Autodesk Inventor part; units mm, degrees
ref_plane "YZ Plane" through (0, 0, 0) normal (1, 0, 0) x (0, 1, 0)
ref_plane "XZ Plane" through (0, 0, 0) normal (0, 1, 0) x (-1, 0, 0)
ref_plane "XY Plane" through (0, 0, 0) normal (0, 0, 1) x (1, 0, 0)
sketch "Sketch1" plane through (0, 0, 0) normal (0, 0, 1) x (1, 0, 0)
  circle A0 centre (-48.3826, -94.0192) radius 2.5
  circle A1 centre (2.8152, 8.6005) radius 2.5
  line L0 (-48.3826, -94.0192) -> (40.5013, 54.4144)
  line L1 (2.8152, 8.6005) -> (32.8522, -42.034)
  line L2 (-2.0828, 38.9998) -> (-2.0828, -39)
  line L3 (-2.0828, -0.0001) -> (69.8745, -0.0001)
  line L4 (7.9172, -0.0001) -> (-0.6834, -5.1021)
  line L5 (2.8152, 8.6005) -> (7.9172, -0.0001)
  line L6 (7.9172, -0.0001) -> (16.5177, 5.1019)
  line L7 (7.9172, -0.0001) -> (-0.6834, -5.1021)
  line L8 (-0.6834, -5.1021) -> (-0.6834, -5.1021)
  line L9 (7.9172, -0.0001) -> (16.5177, 5.1019)
  line L10 (16.5177, 5.1019) -> (16.5177, 5.1019)
  line L11 (7.9172, -0.0001) -> (-0.6622, 5.1374)
  line L12 (7.9172, -0.0001) -> (16.4966, -5.1375)
  line L13 (-48.3826, -94.0192) -> (-43.2452, -85.4397)
  line L14 (-54.6233, -56.9895) -> (-9.7188, -83.8789)
  line L15 (-43.2452, -85.4397) -> (-34.6657, -90.5772)
  line L16 (-43.2452, -85.4397) -> (-51.8246, -80.3023)
  line L17 (-34.6657, -90.5772) -> (16.4966, -5.1375)
  line L18 (-0.6622, 5.1374) -> (-51.8246, -80.3023)
  line L19 (-3.7386, 0) -> (13.452, 10.2217)
  line L20 (-3.7386, 0) -> (13.4203, -10.2749)
  circle A2 centre (6.9172, -34) radius 2.5
  circle A3 centre (6.9172, -34) radius 5
  circle A4 centre (6.9172, 34) radius 2.5
  circle A5 centre (6.9172, 34) radius 4.9998
  line L21 (15.8878, 38.9998) -> (-2.0828, 38.9998)
  line L22 (-2.0828, -39) -> (15.933, -39)
  line L23 (-13.3434, -16.0398) -> (19.6624, -35.8041)
  line L24 (-13.3434, 16.0396) -> (19.6624, 35.8039)
  line L25 (-13.3434, -16.0398) -> (-15.9172, -14.4985)
  line L26 (-2.0828, -0.0001) -> (-26.2435, -0.0001)
  line L27 (-15.9172, -14.4985) -> (-7.2354, -0.0001)
  line L28 (-13.3434, 16.0396) -> (-15.9172, 14.4984)
  line L29 (-15.9172, 14.4984) -> (-7.2354, -0.0001)
  line L30 (13.4203, -10.2749) -> (15.9172, -11.7701)
  line L31 (15.933, -39) -> (15.8878, 38.9998)
  line L32 (13.452, 10.2217) -> (15.9037, 11.6795)
  line L33 (15.9037, 11.6795) -> (6.3124, 27.8097)
  line L34 (15.9172, -11.7701) -> (6.3124, -27.8099)
  line L35 (15.9037, 11.6795) -> (15.9172, -11.7701)
  line L36 (-15.9172, -14.4985) -> (-15.9172, 14.4984)
  line L37 (6.3124, 27.8097) -> (-15.9172, 14.4984)
  circle A6 centre (-48.3826, -94.0192) radius 2.5
  line L38 (-311.4249, 0) -> (127.5863, 0)
  line L39 (-170.3704, -117.2696) -> (-13.4682, 154.4931)
  line L40 (-102.6648, 0) -> (-157.9558, -95.7668)
  line L41 (-157.9558, -95.7668) -> (-48.3826, -94.0192)
  line L42 (-48.3826, -94.0192) -> (-58.3814, -94.1786)
  line L43 (-58.3814, -94.1786) -> (-58.5408, -84.1799)
  line L44 (-58.5408, -84.1799) -> (-58.2219, -104.1774)
  line L45 (-51.8246, -80.3023) -> (-41.5497, -63.1434)
  line L46 (-41.5497, -63.1434) -> (-24.3908, -73.4184)
  line L47 (-58.5408, -84.1799) -> (-78.5383, -84.4989)
  line L48 (-78.5383, -84.4989) -> (-78.2193, -104.4963)
  line L49 (-78.2193, -104.4963) -> (-58.2219, -104.1774)
  line L50 (-58.5408, -84.1799) -> (-51.8246, -80.3023)
  line L51 (-58.2219, -104.1774) -> (-26.2433, -104.1774)
  line L52 (-34.6657, -90.5772) -> (-48.6317, -113.8999)
  circle A7 centre (-48.3828, -94.0194) radius 2.5
  point P0 (0, 0)
  point P1 (6.9172, -21)
  point P2 (-3.7386, 0)
  point P3 (-42.2878, -64.3761)
  point P4 (-42.8097, -104.1774)
  point P5 (-25.129, -74.6511)
  dimension "d0" = 10
  dimension "d1" = 10
  dimension "d2" = 10
  dimension "d3" = 10
  dimension "d4" = 10
  dimension "d5" = 10
  dimension "d6" = 10
  dimension "d7" = 10
  dimension "d8" = 10
  dimension "d9" = 10
  dimension "d10" = 10
  dimension "d11" = 20
  dimension "d12" = 20
  dimension "d13" = 3
  dimension "d14" = 3
  dimension "d20" = 110.582
  dimension "d21" = 10
  dimension "d22" = 10
  dimension "d23" = 20
  dimension "d24" = 20
  dimension "d25" = 20
  dimension "d26" = 121.827
  dimension "d27" = 146.9972
extrude "Extrusion1" add sketch "Sketch1" against normal blind 3 contours A0 L0 L15 L52 L51 L44 L41 | A0 L41 L43 L50 L16 L0 | L16 L18 L14 L0 | L0 L14 L17 L15 | L44 L49 L48 L41 | L41 L48 L47 L43
sketch "Sketch2" plane through (0, 0, -3) normal (0, 0, -1) x (-1, 0, 0)
  line L0 (51.8246, -80.3023) -> (42.2878, -64.3761)
  line L1 (25.129, -74.6511) -> (42.8097, -104.1774)
  line L2 (78.5383, -84.4989) -> (58.5408, -84.1799)
  line L3 (58.5408, -84.1799) -> (51.8246, -80.3023)
  line L4 (42.2878, -64.3761) -> (25.129, -74.6511)
  line L5 (78.5383, -84.4989) -> (78.2193, -104.4963)
  line L6 (58.5408, -84.1799) -> (58.5408, -81.1799)
  line L7 (51.8246, -80.3023) -> (54.3984, -78.761)
  line L8 (42.8097, -104.1774) -> (40.2359, -105.7186)
  line L9 (42.8097, -104.1774) -> (42.7827, -107.1772)
  line L10 (78.5383, -84.4989) -> (78.5383, -81.4989)
  line L11 (78.2193, -104.4963) -> (78.2193, -107.4963)
  line L12 (42.2878, -64.3761) -> (44.8616, -62.8349)
  line L13 (42.2878, -64.3761) -> (25.129, -74.6511)
  line L14 (25.129, -74.6511) -> (22.5551, -76.1923)
  line L15 (78.5383, -81.4989) -> (58.5408, -81.1799)
  line L16 (58.5408, -81.1799) -> (54.3984, -78.761)
  line L17 (54.3984, -78.761) -> (44.8616, -62.8349)
  line L18 (22.5551, -76.1923) -> (40.2359, -105.7186)
  line L19 (40.2359, -105.7186) -> (42.7827, -107.1772)
  line L20 (78.2193, -107.4963) -> (42.7827, -107.1772)
  line L21 (58.5408, -84.1799) -> (58.2219, -104.1774)
  line L22 (51.8246, -80.3023) -> (34.6657, -90.5772)
  circle A0 centre (48.3826, -94.0192) radius 2.5
  circle A1 centre (48.3826, -94.0192) radius 2.5
  line L23 (78.2193, -104.4963) -> (42.8097, -104.1774)
  line L24 (58.2219, -104.1774) -> (42.8097, -104.1774)
  line L25 (78.2193, -104.4963) -> (58.2219, -104.1774)
  point P0 (0, 0)
  dimension "d30" = 3
  dimension "d31" = 3
  dimension "d32" = 3
  dimension "d33" = 3
  dimension "d34" = 3
  dimension "d35" = 3
  dimension "d36" = 3
  dimension "d37" = 3
extrude "Extrusion2" add sketch "Sketch2" along normal blind 20 and the other way blind 3 contours L7 L16 L6 L3 | L0 L12 L17 L7 | L6 L15 L10 L2 | L1 L8 L18 L14 | L25 L23 L24 | L9 L19 L8 | L23 L11 L20 L9
sketch "Sketch3" plane through (0, 0, -3) normal (0, 0, -1) x (-1, 0, 0)
  line L0 (58.5408, -84.1799) -> (51.8246, -80.3023)
  line L1 (51.8246, -80.3023) -> (34.6657, -90.5772)
  line L2 (25.129, -74.6511) -> (42.8097, -104.1774)
  line L3 (42.8097, -104.1774) -> (58.2219, -104.1774)
  line L4 (58.5408, -84.1799) -> (58.2219, -104.1774)
  line L5 (78.2193, -104.4963) -> (42.8097, -104.1774)
  line L6 (42.8097, -104.1774) -> (25.129, -74.6511)
  circle A0 centre (48.3828, -94.0194) radius 2.5
  point P0 (0, 0)
  dimension "d42" = 119.086
extrude "Extrusion3" add sketch "Sketch3" along normal blind 20
sketch "Sketch4" plane through (0, 0, -23) normal (0, 0, -1) x (-1, 0, 0)
  point P0 (0, 0)
sketch "Sketch5" plane through (0, 0, -23) normal (0, 0, -1) x (-1, 0, 0)
  circle A0 centre (48.3828, -94.0194) radius 2.5
  line L0 (44.8616, -62.8349) -> (42.2878, -64.3761)
  line L1 (42.2878, -64.3761) -> (51.8246, -80.3023)
  line L2 (51.8246, -80.3023) -> (34.6657, -90.5772)
  line L3 (34.6657, -90.5772) -> (25.129, -74.6511)
  line L4 (25.129, -74.6511) -> (22.5551, -76.1923)
  line L5 (22.5551, -76.1923) -> (40.2359, -105.7186)
  line L6 (40.2359, -105.7186) -> (42.7827, -107.1772)
  line L7 (42.7827, -107.1772) -> (78.2193, -107.4963)
  line L8 (78.2193, -107.4963) -> (78.2193, -104.4963)
  line L9 (78.2193, -104.4963) -> (58.2219, -104.1774)
  line L10 (58.2219, -104.1774) -> (58.5408, -84.1799)
  line L11 (58.5408, -84.1799) -> (78.5383, -84.4989)
  line L12 (78.5383, -84.4989) -> (78.5383, -81.4989)
  line L13 (78.5383, -81.4989) -> (58.5408, -81.1799)
  line L14 (58.5408, -81.1799) -> (54.3984, -78.761)
  line L15 (54.3984, -78.761) -> (44.8616, -62.8349)
  line L16 (58.5408, -84.1799) -> (58.2219, -104.1774)
  line L17 (58.2219, -104.1774) -> (78.2193, -104.4963)
  line L18 (78.2193, -104.4963) -> (78.5383, -84.4989)
  line L19 (78.5383, -84.4989) -> (58.5408, -84.1799)
  line L20 (34.6657, -90.5772) -> (51.8246, -80.3023)
  line L21 (51.8246, -80.3023) -> (42.2878, -64.3761)
  line L22 (42.2878, -64.3761) -> (25.129, -74.6511)
  line L23 (25.129, -74.6511) -> (34.6657, -90.5772)
  point P0 (0, 0)
extrude "Extrusion4" add sketch "Sketch5" along normal blind 3
sketch "Sketch6" plane through (0, 0, 0) normal (0, 0, 1) x (1, 0, 0)
  line L0 (-42.2878, -64.3761) -> (-25.129, -74.6511)
  line L1 (-33.7084, -69.5136) -> (-49.5228, -95.9232)
  line L2 (-33.7084, -69.5136) -> (-38.8459, -78.093)
  circle A0 centre (-38.8459, -78.093) radius 1.5
  line L3 (-78.5383, -84.4989) -> (-78.2193, -104.4963)
  line L4 (-78.3788, -94.4976) -> (-68.3788, -94.4976)
  circle A1 centre (-68.3788, -94.4976) radius 1.5
  point P0 (0, 0)
  dimension "d47" = 10
  dimension "d48" = 3
  dimension "d56" = 10
  dimension "d57" = 3
extrude "Extrusion5" cut sketch "Sketch6" against normal through all
sketch "Sketch7" plane through (-44.8616, -62.8349, -26) normal (-0.857942, 0.5137465, 0) x (0, 0, 1)
  line L0 (0, 0) -> (26, 0)
  line L1 (26, 0) -> (13, 0)
  line L2 (13, 0) -> (13, -10)
  line L3 (13, -10) -> (26, -10)
  line L4 (26, -10) -> (26, 0)
  circle A0 centre (13, -10) radius 1.5
  point P0 (26, 76.9562)
  dimension "d51" = 13
  dimension "d52" = 10
  dimension "d53" = 3
extrude "Extrusion6" cut sketch "Sketch7" against normal through all contours A0 L3 L2 | L2 L3 A0
sketch "Sketch8" plane through (-58.5408, -81.1799, 0) normal (-0.0159478, 0.9998728, 0) x (0.9998728, 0.0159478, 0)
  line L0 (-20.0478, 3) -> (-20.0478, 23)
  line L1 (-20.0478, 13) -> (-10.0478, 13)
  circle A0 centre (-10.0478, 13) radius 1.5
  point P0 (59.828, 0)
  dimension "d58" = 10
  dimension "d59" = 3
extrude "Extrusion7" cut sketch "Sketch8" against normal through all
fillet "Fillet1" radius 2 5 edges at (-60.501, -107.3368, 0) (-31.3955, -90.9554, 0) (-49.63, -70.798, 0) (-68.5396, -81.3394, 0) (-56.4696, -79.9705, 0)
properties part number "2020_nodes_conn" material "PET Plastic"
For this review, take the finished solid that the model builds, in its own axes (mm). A direction names the side the tool comes from. Round coordinates to 2 decimals unless told otherwise and drop trailing zeros. Loops run counter-clockwise (first coordinate to the right, second up) from the corner with the lowest first, then second, coordinate; pieces in that order, holes last.
(1) Clearance check with flat-ended pins moving along their axes: P1, Ø12, axis at y = -84.5, z = -5.5, coming from the +X side; P2, Ø8, axis at x = -69.5, z = -8.5, coming from the -Y side; P3, Ø3.5, axis at y = -106.5, z = -8, coming from the -X side. State where each tip first meets the part, or that it passes through.
Returned:
P1: stops at x = -23.94
P2: stops at y = -107.45
P3: stops at x = -78.22
(2) Mouldability with a two-part tool opening along Y and no side actions: class faces 1 (the flat face through (-38, -74, -23)), 2 (the flat face through (-56.5, -79.99, -13.83)), 3 (the cylindrical face through (-49.025, -72.667, -11.614)), 4 (the flat face through (-78.538, -83, -13)) as released by +Y, released by -Y, zero draft, split by the parting line, or undercut.
Returned:
face 1: undercut
face 2: released by +Y
face 3: undercut
face 4: zero draft
(3) Wall thickness on line 1 along Z through (x, y) = (-69, -87.5); line 2 along X through (y, z) = (-82, -12.5); line 3 along X through (y, z) = (-80.5, -4.5): over which ranges is each line inside the solid? List them lowest first.
Returned:
line 1: z = -26 to -23, -3 to 0
line 2: x = -78.54 to -69.99, -67.16 to -48.99, -29.53 to -26.03
line 3: x = -57.38 to -51.49, -28.63 to -25.13
(4) We need section A-A (z = -19). Give the boundary of the cut face in (x, y), plus the area to 3 significant figures.
Returned:
outline: (-78.54, -84.5) - (-58.54, -84.18) - (-58.22, -104.18) - (-78.22, -104.5) - (-78.22, -107.5) - (-42.78, -107.18) - (-40.24, -105.72) - (-22.56, -76.19) - (-25.13, -74.65) - (-34.67, -90.58) - (-51.82, -80.3) - (-42.29, -64.38) - (-44.86, -62.83) - (-54.4, -78.76) - (-58.54, -81.18) - (-78.54, -81.5) - close; hole circle Ø5 at (-48.38, -94.02)
area: 739 mm2
(5) We need section B-B (x = -39.5). State how many separate pieces and enclosed holes the cut face has, plus the area to 3 significant figures.
Returned:
separate pieces: 3
enclosed holes: 0
area: 549 mm2
(6) Tool access review of faces 5 (the flat face through (-78.219, -106, -13)), 6 (the cylindrical face through (-68.43, -81.94, -0.57)): name each direction out of +Z, -Z, +X, -X, +Y, -Y from which nothing blocks a thin tool from reaching the whole face with its end or side.
Returned:
face 5: +Z, -Z, -X, -Y
face 6: +Z, -X, +Y
